from build123d import *

# Parameters (mm, degrees)
ESQUISSE1_R        = 2.5
BOSS_EXTRU_1_DEPTH = 5
ESQUISSE2_R        = 5
BOSS_EXTRU_2_DEPTH = 36
CONG_1_R           = 3


with BuildPart() as part:
    # Esquisse1 → Boss.-Extru.1 (new, symmetric)
    with BuildSketch(Plane.XY):
        with BuildLine():
            Line((5, 10), (5, -10))
            ThreePointArc((5, -10), (0, -15), (-5, -10))
            Line((-5, -10), (-5, 10))
            ThreePointArc((-5, 10), (0, 15), (5, 10))
        make_face()
        with Locations((0, 10)):
            Circle(ESQUISSE1_R, mode=Mode.SUBTRACT)
        with Locations((0, -10)):
            Circle(ESQUISSE1_R, mode=Mode.SUBTRACT)
    extrude(amount=BOSS_EXTRU_1_DEPTH, both=True)

    # Esquisse2 → Boss.-Extru.2 (add)
    with BuildSketch(Plane(origin=(5, 0, 0), x_dir=(0, 0, -1), z_dir=(1, 0, 0))):
        with Locations((0, 5)):
            Circle(ESQUISSE2_R)
    extrude(amount=BOSS_EXTRU_2_DEPTH)

    # Congé1
    cong_1_edges = [part.edges().sort_by_distance(p)[0] for p in [
        (41, 5, 5),
    ]]
    fillet(cong_1_edges, radius=CONG_1_R)


solid = part.part
Geometry: final body of the model. Coordinates: model frame, mm. A direction names the side the tool comes from. Round coordinates to 2 decimals unless told otherwise and drop trailing zeros. Order: outer loops, then holes, each group sorted by start corner. A loop starts at its lowest first (then second) coordinate and runs counter-clockwise, first axis right, second up.
Q1. Section C-C, the plane y = -6.5. Output: boundary loops of the cut face in (x, z).
Result sheet:
outline: (-5, -5) - (5, -5) - (5, 5) - (-5, 5) - close
Q2. Section A-A, the plane x = 0. Output: boundary loops of the cut face in (y, z).
Result sheet:
outline: (-15, -5) - (-12.5, -5) - (-12.5, 5) - (-15, 5) - close; (-7.5, -5) - (7.5, -5) - (7.5, 5) - (-7.5, 5) - close; (12.5, -5) - (15, -5) - (15, 5) - (12.5, 5) - close
Q3. Pin query (flat end, axial travel): pin 1 (6 mm diameter, centred on x = 31, z = -3, fed in from -Y); pin 2 (1.5 mm diameter, centred on x = 23.5, z = 4, fed in from +Y); pin 3 (2 mm diameter, centred on y = -6, z = -1, fed in from +X). Return the tip coordinate at first contact, or that it passes through.
Result sheet:
pin 1: stops at y = 0
pin 2: stops at y = 8.8
pin 3: stops at x = 5
Q4. Access query for faces 1 (the face through (5, 9, -4)), 2 (the face through (21.27, 0.12, 1.08)), 3 (the face through (5, 9, 4)). Directions: +Z, -Z, +X, -X, +Y, -Y. A direction counts if a zero-diameter tool reaches every point of the face in a straight line with its end or side. Return the directions, or none.
Result sheet:
face 1: -Z, +X, +Y
face 2: +X
face 3: +Z, +X, +Y
Q5. Section B-B, the plane y = 11. Output: boundary loops of the cut face in (x, z).
Result sheet:
outline: (-4.9, -5) - (-2.29, -5) - (-2.29, 5) - (-4.9, 5) - close; (2.29, -5) - (4.9, -5) - (4.9, 5) - (2.29, 5) - close
Q6. Section D-D, the plane x = 8. Output: boundary loops of the cut face in (y, z).
Result sheet:
outline: circle Ø10 at (5, 0)
Q7. Mould query, pull axis Y, two halves, no side actions, for faces 4 (the face through (5, -4, 0)), 5 (the face through (0, 15, 0)), 6 (the face through (-0.54, 7.56, -0.07)). Classes: released by +Y, released by -Y, zero draft, split by the parting line, or undercut.
Result sheet:
face 4: zero draft
face 5: released by +Y
face 6: undercut
Q8. Material intervals for probe 1 along Y at (x, z) = (0, 0.75); probe 2 along Y at (x, z) = (0.5, 2); probe 3 along X at (y, z) = (-3.5, 1.25), sorted ascending.
Result sheet:
probe 1: y = -15 to -12.5, -7.5 to 7.5, 12.5 to 15
probe 2: y = -14.97 to -12.45, -7.55 to 7.55, 12.45 to 14.97
probe 3: x = -5 to 5
